from build123d import *

# Parameters (mm, degrees)
F0_W     = 30
F0_H     = 30
F0_R     = 1.25
F0_R_2   = 2.05
F1_DEPTH = 6
F2_R     = 4.5
F3_DEPTH = 3
F4_R     = 3


with BuildPart() as f1:
    # F0 (on Top) → F1 (new body)
    with BuildSketch(Plane.XY):
        Rectangle(F0_W, F0_H)
        with Locations((-12, -10)):
            Circle(F0_R, mode=Mode.SUBTRACT)
        with Locations((12, -10)):
            Circle(F0_R, mode=Mode.SUBTRACT)
        with Locations((0, -7)):
            Circle(F0_R_2, mode=Mode.SUBTRACT)
        with Locations((-12, 10)):
            Circle(F0_R, mode=Mode.SUBTRACT)
        with Locations((0, 7)):
            Circle(F0_R_2, mode=Mode.SUBTRACT)
        with Locations((12, 10)):
            Circle(F0_R, mode=Mode.SUBTRACT)
    extrude(amount=F1_DEPTH)

    # F2 (on face) → F3 (cut)
    with BuildSketch(Plane.XY.offset(6)):
        with Locations((0, 7)):
            Circle(F2_R)
        with Locations((0, -7)):
            Circle(F2_R)
    extrude(amount=-F3_DEPTH, mode=Mode.SUBTRACT)

    # F4
    f4_edges = [f1.edges().sort_by_distance(p)[0] for p in [
        (15, -15, 3),
        (15, 15, 3),
        (-15, -15, 3),
        (-15, 15, 3),
    ]]
    fillet(f4_edges, radius=F4_R)


solid = f1.part
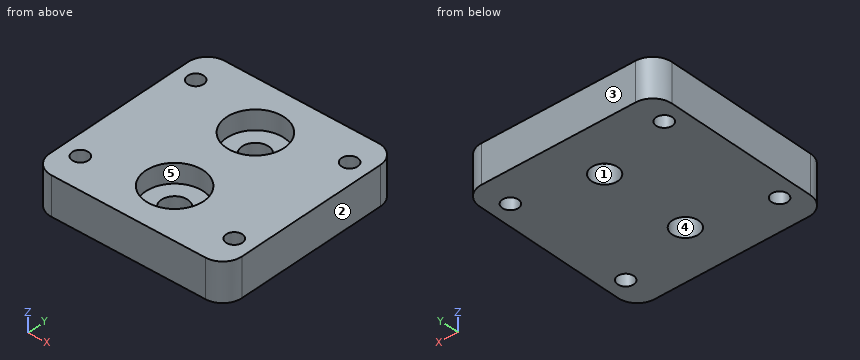
Geometry check sheet. Reference: the model listing, model coordinates, mm. Face numbers are marked on the shaded views. A direction names the side the tool comes from. Coordinates: 2 decimals unless noted, no trailing zeros. Order: outer loops, then holes, each group sorted by start corner. A loop starts at its lowest first (then second) coordinate and runs counter-clockwise, first axis right, second up. Notation, with made-up numbers: (34, 89) -> (51, 89) arc R25 ccw to (51, 114) -> close; hole circle Ø11 at (33.5, -25). An arc over 180 degrees is marked (long way). Use a Markdown table: item, result. Add a question column.
1. Cross-section at B-B (z = 1.1). Enter the section's corners in (x, y), and give its area (3 significant figures).
2. Cross-section at C-C (y = 10.5). Enter the section's corners in (x, z), and give its area (3 significant figures).
3. Cross-section at A-A (y = 7). Enter the section's corners in (x, z).
4. Mould release check, pull along Y, two halves, no side actions. Record for the marked faces 1, 2 and 3: pulls with the +Y half, pulls with the -Y half, needs draft (parallel to the pull), parting line crosses it, or undercut.
5. Set-up check for the marked faces 4 and 5: record each of +Z, -Z, +X, -X, +Y, -Y from which the full face is reachable in a straight line by a thin tool's end or side.
6. Go/stop test with flat-tipped pins: pin 1 Ø10.5 at (x, y) = (0, 7) entering from +Z; pin 2 Ø4.5 at (x, y) = (0.5, -6) entering from +Z. Record where each tip stops, or that it passes through.
7. Material ranges on L1, parallel to Y at x = 0, z = 0.7; L2, parallel to Y at x = -12, z = 1.6; L3, parallel to X at y = 7, z = 1.95, recorded low to high.
8. Cross-section at D-D (z = 4.9). Enter the section's corners in (x, y), and give its area (3 significant figures).
Filled sheet:
| question | item | result |
|---|---|---|
| 1 | outline | (-15, -12) arc R3 ccw to (-12, -15) -> (12, -15) arc R3 ccw to (15, -12) -> (15, 12) arc R3 ccw to (12, 15) -> (-12, 15) arc R3 ccw to (-15, 12) -> close; hole circle Ø2.5 at (-12, -10); hole circle Ø2.5 at (-12, 10); hole circle Ø4.1 at (0, -7); hole circle Ø4.1 at (0, 7); hole circle Ø2.5 at (12, -10); hole circle Ø2.5 at (12, 10) |
| 1 | area | 846 mm2 |
| 2 | outline | (-15, 0) -> (-13.15, 0) -> (-13.15, 6) -> (-15, 6) -> close; (-10.85, 0) -> (10.85, 0) -> (10.85, 6) -> (2.83, 6) -> (2.83, 3) -> (-2.83, 3) -> (-2.83, 6) -> (-10.85, 6) -> close; (13.15, 0) -> (15, 0) -> (15, 6) -> (13.15, 6) -> close |
| 2 | area | 136 mm2 |
| 3 | outline | (-15, 0) -> (-2.05, 0) -> (-2.05, 3) -> (-4.5, 3) -> (-4.5, 6) -> (-15, 6) -> close; (2.05, 0) -> (15, 0) -> (15, 6) -> (4.5, 6) -> (4.5, 3) -> (2.05, 3) -> close |
| 4 | face 1 | undercut |
| 4 | face 2 | needs draft |
| 4 | face 3 | pulls with the +Y half |
| 5 | face 4 | +Z, -Z |
| 5 | face 5 | +Z |
| 6 | pin 1 | z = 6 |
| 6 | pin 2 | z = 3 |
| 7 | L1 | -15 to -9.05, -4.95 to 4.95, 9.05 to 15 |
| 7 | L2 | -15 to -11.25, -8.75 to 8.75, 11.25 to 15 |
| 7 | L3 | -15 to -2.05, 2.05 to 15 |
| 8 | outline | (-15, -12) arc R3 ccw to (-12, -15) -> (12, -15) arc R3 ccw to (15, -12) -> (15, 12) arc R3 ccw to (12, 15) -> (-12, 15) arc R3 ccw to (-15, 12) -> close; hole circle Ø2.5 at (-12, -10); hole circle Ø2.5 at (-12, 10); hole circle Ø9 at (0, -7); hole circle Ø9 at (0, 7); hole circle Ø2.5 at (12, -10); hole circle Ø2.5 at (12, 10) |
| 8 | area | 745 mm2 |
